Check sheet for the modelled part. Datum: model origin and axes. Units: mm. A direction names the side the tool comes from. Round coordinates to 2 decimals unless told otherwise and drop trailing zeros. Order: outer loops, then holes, each group sorted by start corner. A loop starts at its lowest first (then second) coordinate and runs counter-clockwise, first axis right, second up. Notation, with made-up numbers: M -17.5,50.5 L -10.5,50.5 A12 ccw -10.5,64.5 Z; hole C 60,-9 d1. An arc over 180 degrees is marked long. One line per item, written item: value. Start each with the question number.
(1) Release check for a two-part mould opening along Z. For faces 1 (the face through (-56, 0, -24.5)), 2 (the face through (-54, 0, 16.872)), 3 (the face through (-5, -11, 0)), 4 (the face through (-56, 0, -17)) record: released by +Z, released by -Z, zero draft, split by the parting line, or undercut.
(2) Cross-section at B-B, the plane x = -65. Enter the section's corners in (y, z).
(3) Depth check by flat-ended pin: pin 1 Ø14.5 at (x, z) = (-50.5, -11.5) entering from -Y; pin 2 Ø1 at (x, z) = (-43, 17.5) entering from +Y. Enter the tip coordinate at first touch or a pass-through.
(4) Cross-section at A-A, the plane y = -14.5. Enter the section's corners in (x, z), and give its area (3 significant figures).
(5) Cross-section at C-C, the plane z = 7.5. Enter the section's corners in (x, y), and give its area (3 significant figures).
(6) Thickness scan on L1, parallel to X at y = -5, z = 9; L2, parallel to Z at x = -35, y = -1; L3, parallel to Y at x = -104, z = 16.5. Record the ranges inside material, lowest first.
(7) Access from +Z, -Z, +X, -X, +Y, -Y to the whole of each face (thin tool, end or side, straight path). Record for faces 5 (the face through (-12.5, 0, 0)), 6 (the face through (-2.465, -2.615, 0.751)), 7 (the face through (-105, -11, 0)), 8 (the face through (-56, 0, 24.5)), 9 (the face through (-105, 11, 0)).
(8) Cross-section at D-D, the plane y = -5.5. Enter the section's corners in (x, z).
Autodesk Inventor part; units mm, degrees
ref_plane "YZ Plane" through (0, 0, 0) normal (1, 0, 0) x (0, 1, 0)
ref_plane "XZ Plane" through (0, 0, 0) normal (0, 1, 0) x (-1, 0, 0)
ref_plane "XY Plane" through (0, 0, 0) normal (0, 0, 1) x (1, 0, 0)
sketch "Sketch1" plane through (0, 0, 0) normal (0, 1, 0) x (-1, 0, 0)
  point P0 (0, 0)
sketch "Sketch2" plane through (0, 0, 0) normal (0, 0, 1) x (1, 0, 0)
  line L0 (0, 0) -> (0, 24.5)
  line L1 (0, 24.5) -> (-5, 24.5)
  line L2 (-5, 24.5) -> (-5, 2.5)
  line L3 (-5, 2.5) -> (-105, 2.5)
  line L4 (-105, 2.5) -> (-105, 24.5)
  line L5 (-105, 24.5) -> (-110, 24.5)
  line L6 (-110, 24.5) -> (-110, 0)
  line L7 (-110, 0) -> (0, 0)
  line L8 (-105, 2.5) -> (-5, 2.5)
  line L9 (-5, 2.5) -> (-5, -2.5)
  line L10 (-5, -2.5) -> (-105, -2.5)
  line L11 (-105, -2.5) -> (-105, 2.5)
  point P0 (-5, 2.5)
  dimension "d0" = 24.5
  dimension "d1" = 5
  dimension "d2" = 22
  dimension "d3" = 100
  dimension "d4" = 5
  dimension "d6" = 5
revolve "Revolution1" add sketch "Sketch2" angle 360 about axis through (-110, 0, 0) along (1, 0, 0) contours L7 L9 L2 L1 L0 | L7 L11 L3 L9 | L7 L6 L5 L4 L11
extrude "Extrusion1" add sketch "Sketch2" along normal mid plane 49 contours L9 L10 L11 L7 | L7 L11 L3 L9
sketch "Sketch3" plane through (-105, 2.5, -24.5) normal (0, 1, 0) x (1, 0, 0)
  line L0 (100, 0) -> (0, 0)
  line L1 (100, -48.8721) -> (100, -0.1279)
  line L2 (0, 0) -> (100, 0)
  line L3 (100, 0) -> (100, -48.8721)
  line L4 (100, -48.8721) -> (0, -48.8721)
  line L5 (0, -48.8721) -> (0, 0)
  line L6 (7.5, -7.5) -> (92.5, -7.5)
  line L7 (92.5, -7.5) -> (92.5, -41.3721)
  line L8 (92.5, -41.3721) -> (7.5, -41.3721)
  line L9 (7.5, -41.3721) -> (7.5, -7.5)
  point P0 (105, -24.5)
  dimension "d9" = 7.5
extrude "Extrusion2" cut sketch "Sketch3" against normal mid plane 20 contours L6 L7 L8 L9
sketch "Sketch4" plane through (0, 0, 0) normal (1, 0, 0) x (0, 1, 0)
  circle A0 centre (-5, 0) radius 2.5
  point P0 (0, 0)
  dimension "d13" = 5
  dimension "d16" = 5
extrude "Extrusion3" cut sketch "Sketch4" against normal blind 10
properties part number "electronicsbay" material "ABS Plastic"
Values found:
1. face 1: released by -Z
1. face 2: undercut
1. face 3: zero draft
1. face 4: undercut
2. outline: M -2.5,-24.5 L 2.5,-24.5 L 2.5,-17 L -2.5,-17 Z; M -2.5,16.87 L 2.5,16.87 L 2.5,24.5 L -2.5,24.5 Z
3. pin 1: y = -2.5
3. pin 2: y = 2.5
4. outline: M -110,-19.75 L -105,-19.75 L -105,19.75 L -110,19.75 Z; M -5,-19.75 L 0,-19.75 L 0,19.75 L -5,19.75 Z
4. area: 395 mm^2
5. outline: M -110,-23.32 L -105,-23.32 L -105,-2.5 L -97.5,-2.5 L -97.5,2.5 L -105,2.5 L -105,23.32 L -110,23.32 Z; M -12.5,-2.5 L -5,-2.5 L -5,-23.32 L 0,-23.32 L 0,23.32 L -5,23.32 L -5,2.5 L -12.5,2.5 Z
5. area: 541 mm^2
6. L1: -110 to -105, -5 to 0
6. L2: -24.5 to -17, 16.87 to 24.5
6. L3: -2.5 to 2.5
7. face 5: +Y, -Y
7. face 6: +X
7. face 7: +Z, -Z, -Y
7. face 8: +Z, +X, -X, +Y, -Y
7. face 9: +Z, -Z, +Y
8. outline: M -110,-23.87 L -105,-23.87 L -105,23.87 L -110,23.87 Z; M -5,-23.87 L 0,-23.87 L 0,-2.45 L -5,-2.45 Z; M -5,2.45 L 0,2.45 L 0,23.87 L -5,23.87 Z
